from build123d import *

# Parameters (mm, degrees)
BOSS_EXTRUDE1_DEPTH = 4
CUT_EXTRUDE1_DEPTH  = 55.260943597


with BuildPart() as part:
    # Sketch1 → Boss-Extrude1 (new body)
    with BuildSketch(Plane.XY):
        with BuildLine():
            Line((0, 7.050779416), (0, 41))
            ThreePointArc((0, 41), (1.464466094, 44.535533906), (5, 46))
            Line((5, 46), (23.5, 46))
            ThreePointArc((23.5, 46), (27.035533906, 44.535533906), (28.5, 41))
            Line((28.5, 41), (28.5, 7.050779416))
            ThreePointArc((28.5, 7.050779416), (27.385023171, 3.903305038), (24.537362015, 2.159575061))
            Line((24.537362015, 2.159575061), (17.25, 0))
            Line((17.25, 0), (11.25, 0))
            Line((11.25, 0), (3.962637985, 2.159575061))
            ThreePointArc((3.962637985, 2.159575061), (1.114976829, 3.903305038), (0, 7.050779416))
        make_face()
        with BuildLine():
            Line((10.25, 42.5), (18.25, 42.5))
            ThreePointArc((18.25, 42.5), (26, 34.75), (18.25, 27))
            Line((18.25, 27), (10.25, 27))
            ThreePointArc((10.25, 27), (2.5, 34.75), (10.25, 42.5))
        make_face(mode=Mode.SUBTRACT)
    extrude(amount=BOSS_EXTRUDE1_DEPTH)

    # Sketch2 → Cut-Extrude1 (cut, through all)
    with BuildSketch(Plane.ZY):
        Polygon((0, 0), (0, 7.050779416), (0.7, 0), align=None)
        Polygon((4, 7.050779416), (3.3, 0), (4, 0), align=None)
    extrude(amount=-CUT_EXTRUDE1_DEPTH, mode=Mode.SUBTRACT)


solid = part.part
Read the model definition and answer for the solid it produces. Units are mm, in the model's axes. A direction names the side the tool comes from. Round coordinates to 2 decimals unless told otherwise and drop trailing zeros. Order: outer loops, then holes, each group sorted by start corner. A loop starts at its lowest first (then second) coordinate and runs counter-clockwise, first axis right, second up.
1) The part is cut by section B-B on y = 34.75. Write down the section's boundary in (x, z), plus the area to 3 significant figures.
2) The part is cut by section D-D on x = 6.25. Write down the section's boundary in (y, z).
3) Straight lines are drawn through the part: L1, parallel to Y at x = 11.75, z = 3.2; L2, parallel to Y at x = 10, z = 2.7; L3, parallel to X at y = 35.5, z = 3.4. For each, find the intervals that lie inside material, in ascending order.
4) For faces 5 (the face through (2.5, 34.6, 2)), 6 (the face through (14.05, 4.358, 3.733)), determine the directions among +Z, -Z, +X, -X, +Y, -Y from which every point of the face is accessible in a straight line to the end or side of a thin tool.
5) The part is cut by section C-C on x = 22.5. Write down the section's boundary in (y, z).
6) The part is cut by section A-A on z = 2.65. Write down the section's boundary in (x, y).
7) Flat-ended cylindrical pins translate along their axes: pin 1 (2 mm diameter, centred on y = 5, z = 1, fed in from +X); pin 2 (1.5 mm diameter, centred on x = 24, z = 3, fed in from -Y); pin 3 (3 mm diameter, centred on x = 3, y = 5.5, fed in from -Z). Find the tip coordinate at first contact, or state that the pin passes through.
8) The mould has two halves that part along X. Classify faces 1 (the face through (7.657, 1.065, 1.979)), 2 (the face through (14, 42.5, 2)), 3 (the face through (14, 22, 4)), 4 (the face through (20.945, 1.095, 1.979)): released by +X, released by -X, zero draft, split by the parting line, or undercut.
Resolved:
1. outline: (0, 0) - (2.5, 0) - (2.5, 4) - (0, 4) - close; (26, 0) - (28.5, 0) - (28.5, 4) - (26, 4) - close
1. area: 20.0 mm2
2. outline: (1.48, 0.55) - (7.05, 0) - (28.11, 0) - (28.11, 4) - (7.05, 4) - (1.48, 3.45) - close; (41.39, 0) - (46, 0) - (46, 4) - (41.39, 4) - close
3. L1: y = 0 to 27, 42.5 to 46
3. L2: y = 0.37 to 27, 42.5 to 46
3. L3: x = 0 to 2.54, 25.96 to 28.5
4. face 5: +Z, -Z
4. face 6: +Z, +X, -X, -Y
5. outline: (1.56, 0.55) - (7.05, 0) - (28.27, 0) - (28.27, 4) - (7.05, 4) - (1.56, 3.45) - close; (41.23, 0) - (46, 0) - (46, 4) - (41.23, 4) - close
6. outline: (0, 7.05) arc R5 ccw to (3.96, 2.16) - (11.25, 0) - (17.25, 0) - (24.54, 2.16) arc R5 ccw to (28.5, 7.05) - (28.5, 41) arc R5 ccw to (23.5, 46) - (5, 46) arc R5 ccw to (0, 41) - close; hole (10.25, 27) - (18.25, 27) arc R7.75 ccw to (18.25, 42.5) - (10.25, 42.5) arc R7.75 ccw to start
7. pin 1: stops at x = 28.39
7. pin 2: stops at y = 1.78
7. pin 3: stops at z = 0.01
8. face 1: released by -X
8. face 2: undercut
8. face 3: zero draft
8. face 4: released by +X
